Here's how the part is built. I have some questions about the finished solid (model axes, mm). Coordinates: 2 decimals unless noted, no trailing zeros. Order: outer loops, then holes, each group sorted by start corner. A loop starts at its lowest first (then second) coordinate and runs counter-clockwise, first axis right, second up. Notation, with made-up numbers: (-27, -39) - (-21, -39) arc R31 ccw to (-21, -4) - close; hole circle Ø9 at (-35, 40). An arc over 180 degrees is marked (long way). Answer in a Markdown table with one row per item. Add a question column.
Item 1: If I drill on line 1 along Z through (x, y) = (0, 3.5); line 2 along X through (y, z) = (1.4, -50.5); line 3 along Z through (x, y) = (-71, 0.55), over which ranges is the centre line in solid material (lowest first)? Write a range as from..to.
Item 2: I want a section at C-C (y = 3.7). Please give me the cut outline in (x, z), plus the area to 3 significant figures.
Item 3: I want a section at B-B (z = 0). Please give me the cut outline in (x, y), plus the area to 3 significant figures.
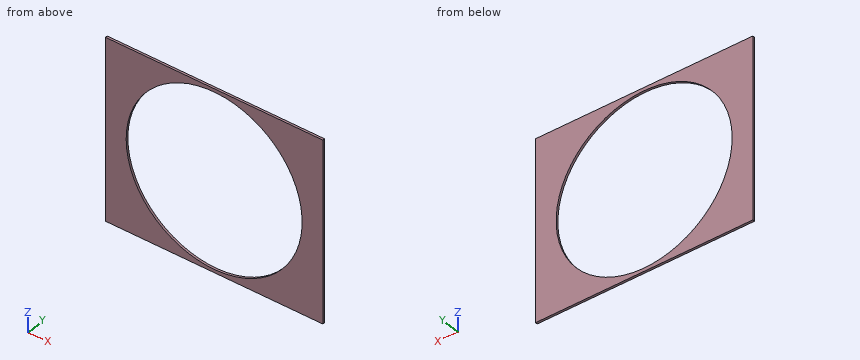
Autodesk Inventor part; units mm, degrees
ref_plane "YZ Plane" through (0, 0, 0) normal (1, 0, 0) x (0, 1, 0)
ref_plane "XZ Plane" through (0, 0, 0) normal (0, 1, 0) x (-1, 0, 0)
ref_plane "XY Plane" through (0, 0, 0) normal (0, 0, 1) x (1, 0, 0)
sketch "Skizze1" plane through (0, 0, 0) normal (0, 1, 0) x (-1, 0, 0)
  line L0 (-250, 210) -> (250, 210)
  line L1 (250, 210) -> (250, -210)
  line L2 (250, -210) -> (-250, -210)
  line L3 (-250, -210) -> (-250, 210)
  line L4 (-250, 210) -> (250, -210) construction
  line L5 (250, 210) -> (-250, -210) construction
  circle A0 centre (0, 0) radius 202.5
  dimension "d0" = 500
  dimension "d1" = 420
  dimension "d2" = 405
extrude "Extrusion1" add sketch "Skizze1" along normal blind 5
properties part number "Boden_drehscheibe" material "Holz (Birke)"
Values follow:
| question | item | result |
|---|---|---|
| 1 | line 1 | z = -210..-202.5, 202.5..210 |
| 1 | line 2 | x = -250..-196.1, 196.1..250 |
| 1 | line 3 | z = -210..-189.65, 189.65..210 |
| 2 | outline | (-250, -210) - (250, -210) - (250, 210) - (-250, 210) - close; hole circle Ø405 at (0, 0) |
| 2 | area | 81,200 mm^2 |
| 3 | outline | (-250, 0) - (-202.5, 0) - (-202.5, 5) - (-250, 5) - close; (202.5, 0) - (250, 0) - (250, 5) - (202.5, 5) - close |
| 3 | area | 475 mm^2 |
